Read the model definition and answer for the solid it produces. Units are mm, in the model's axes. A direction names the side the tool comes from. Round coordinates to 2 decimals unless told otherwise and drop trailing zeros. Order: outer loops, then holes, each group sorted by start corner. A loop starts at its lowest first (then second) coordinate and runs counter-clockwise, first axis right, second up. Notation, with made-up numbers: (48.25, 67) -> (68.25, 67) arc R18 ccw to (68.25, 83) -> close; hole circle Ø11 at (-8, 14.5). An arc over 180 degrees is marked (long way). Answer as a JSON object with one key per item and string values. Group by question number.
Item 1: Consider probe 1 along Y at (x, z) = (14, -0.75); probe 2 along X at (y, z) = (-0.25, -14.5); probe 3 along X at (y, z) = (-0.5, 1.75). Determine where each line is inside the solid, lowest interval first. Write a range as from..to.
Item 2: Section D-D, the plane z = -10 is taken. Write down the section's boundary in (x, y).
Item 3: The mould has two halves that part along Z. Classify faces 1 (the flat face through (0, -7.45, 0)), 2 (the flat face through (5, -5, -15.8)), 3 (the flat face through (-0.41, -3.56, -9.54)): pulls with the +Z half, pulls with the -Z half, needs draft (parallel to the pull), parting line crosses it, or undercut.
Item 4: Given P1, Ø0.5, axis at x = 5.5, z = -14.5, coming from the +Y side; P2, Ø9, axis at x = 1.5, z = -7, coming from the -Y side; P3, Ø4.5, axis at x = 1.5, z = -0.5, coming from the -Y side, each flat-ended and moving along its own axis, determine where each tip first touches the part or whether it passes through.
Item 5: For faces 4 (the flat face through (4.7, -5, -15)), 5 (the flat face through (0.1, -6.1, 2.5)), 6 (the cylindrical face through (-8.4, 0.1, -1.5)), determine the directions among +Z, -Z, +X, -X, +Y, -Y from which every point of the face is accessible in a straight line to the end or side of a thin tool.
Item 6: Section C-C, the plane x = 14 is taken. Write down the section's boundary in (y, z), plus the area to 3 significant figures.
Item 7: Section A-A, the plane z = -2.5 is taken. Write down the section's boundary in (x, y), plus the area to 3 significant figures.
Item 8: Section B-B, the plane y = -10 is taken. Write down the section's boundary in (x, z).
from build123d import *

# Parameters (mm, degrees)
SKETCH1_R                = 1.6
BOSS_EXTRUDE1_DEPTH      = 2
BOSS_EXTRUDE2_DEPTH      = 1
BOSS_EXTRUDE2_DEPTH_BACK = 15.2
BOSS_EXTRUDE3_START      = -9.8
BOSS_EXTRUDE3_DEPTH      = 1
BOSS_EXTRUDE4_START      = 5.2
BOSS_EXTRUDE4_DEPTH      = 0.5
BOSS_EXTRUDE6_DEPTH      = 1
SKETCH6_R                = 1
BOSS_EXTRUDE7_DEPTH      = 8.8
FILLET1_R                = 1


with BuildPart() as part:
    # Sketch1 → Boss-Extrude1 (new, symmetric)
    with BuildSketch(Plane.XY):
        with BuildLine():
            Line((-14.4, 7.45), (14.4, 7.45))
            ThreePointArc((14.4, 7.45), (16.521320344, 6.571320344), (17.4, 4.45))
            Line((17.4, 4.45), (17.4, -4.45))
            ThreePointArc((17.4, -4.45), (16.521320344, -6.571320344), (14.4, -7.45))
            Line((14.4, -7.45), (-14.4, -7.45))
            ThreePointArc((-14.4, -7.45), (-16.521320344, -6.571320344), (-17.4, -4.45))
            Line((-17.4, -4.45), (-17.4, 4.45))
            ThreePointArc((-17.4, 4.45), (-16.521320344, 6.571320344), (-14.4, 7.45))
        make_face()
        with Locations((14, 0)):
            Circle(SKETCH1_R, mode=Mode.SUBTRACT)
        with Locations(Location((-14, 0, 0), (0, 0, 180))):
            Circle(SKETCH1_R, mode=Mode.SUBTRACT)
        with BuildLine():
            Line((-4.15, 4.25), (-0.808290377, 4.25))
            Line((-0.808290377, 4.25), (0, 2.85))
            Line((0, 2.85), (0.808290377, 4.25))
            Line((0.808290377, 4.25), (4.15, 4.25))
            ThreePointArc((4.15, 4.25), (8.4, 0), (4.15, -4.25))
            Line((4.15, -4.25), (0.808290377, -4.25))
            Line((0.808290377, -4.25), (0, -2.85))
            Line((0, -2.85), (-0.808290377, -4.25))
            Line((-0.808290377, -4.25), (-4.15, -4.25))
            ThreePointArc((-4.15, -4.25), (-8.4, 0), (-4.15, 4.25))
        make_face(mode=Mode.SUBTRACT)
    extrude(amount=BOSS_EXTRUDE1_DEPTH, both=True)

    # Sketch2 → Boss-Extrude2 (add, two sides: drawn at the far end of the back side and taken through both)
    with BuildSketch(Plane.XY.offset(2).offset(-BOSS_EXTRUDE2_DEPTH_BACK)):
        with BuildLine():
            Line((-4.15, 6.1), (4.15, 6.1))
            ThreePointArc((4.15, 6.1), (10.25, 0), (4.15, -6.1))
            Line((4.15, -6.1), (-4.15, -6.1))
            ThreePointArc((-4.15, -6.1), (-10.25, 0), (-4.15, 6.1))
        make_face()
        with BuildLine():
            Line((0.808290377, 4.25), (0, 2.85))
            Line((0, 2.85), (-0.808290377, 4.25))
            Line((-0.808290377, 4.25), (-4.15, 4.25))
            ThreePointArc((-4.15, 4.25), (-8.4, 0), (-4.15, -4.25))
            Line((-4.15, -4.25), (-0.808290377, -4.25))
            Line((-0.808290377, -4.25), (0, -2.85))
            Line((0, -2.85), (0.808290377, -4.25))
            Line((0.808290377, -4.25), (4.15, -4.25))
            ThreePointArc((4.15, -4.25), (8.4, 0), (4.15, 4.25))
            Line((4.15, 4.25), (0.808290377, 4.25))
        make_face(mode=Mode.SUBTRACT)
    extrude(amount=BOSS_EXTRUDE2_DEPTH + BOSS_EXTRUDE2_DEPTH_BACK)

    # Sketch3 → Boss-Extrude3 (add)
    with BuildSketch(Plane.XY.offset(3).offset(BOSS_EXTRUDE3_START)):
        with BuildLine():
            Line((0.808290377, 4.25), (0, 2.85))
            Line((0, 2.85), (-0.808290377, 4.25))
            Line((-0.808290377, 4.25), (-4.15, 4.25))
            ThreePointArc((-4.15, 4.25), (-8.4, 0), (-4.15, -4.25))
            Line((-4.15, -4.25), (-0.808290377, -4.25))
            Line((-0.808290377, -4.25), (0, -2.85))
            Line((0, -2.85), (0.808290377, -4.25))
            Line((0.808290377, -4.25), (4.15, -4.25))
            ThreePointArc((4.15, -4.25), (8.4, 0), (4.15, 4.25))
            Line((4.15, 4.25), (0.808290377, 4.25))
        make_face()
    extrude(amount=BOSS_EXTRUDE3_DEPTH)



with BuildPart() as body_2:
    # Sketch4 → Boss-Extrude4 (new, symmetric)
    with BuildSketch(Plane(origin=(0, 0, 0), x_dir=(0, 0, -1), z_dir=(1, 0, 0)).offset(BOSS_EXTRUDE4_START)):
        with BuildLine():
            Line((13.2, 1), (15.8, 1))
            Line((15.8, 1), (15.8, -10.62))
            ThreePointArc((15.8, -10.62), (14.8, -11.62), (13.8, -10.62))
            Line((13.8, -10.62), (13.8, -1))
            Line((13.8, -1), (13.2, -1))
            Line((13.2, -1), (13.2, 1))
        make_face()
    boss_extrude4 = extrude(amount=BOSS_EXTRUDE4_DEPTH, both=True)


with BuildPart() as part_1:
    add(part.part)

    add(body_2.part)  # Boss-Extrude6 merges body 2
    # Sketch5 → Boss-Extrude6 (add)
    with BuildSketch(Plane(origin=(0, 0, -13.2), x_dir=(-1, 0, 0), z_dir=(0, 0, -1))):
        with BuildLine():
            Line((4.15, 6.1), (-4.15, 6.1))
            ThreePointArc((-4.15, 6.1), (-10.25, 0), (-4.15, -6.1))
            Line((-4.15, -6.1), (4.15, -6.1))
            ThreePointArc((4.15, -6.1), (10.25, 0), (4.15, 6.1))
        make_face()
    extrude(amount=-BOSS_EXTRUDE6_DEPTH)

    # Mirror2: Boss-Extrude4 across plane
    add(boss_extrude4.mirror(Plane(origin=(0, 0, 0), x_dir=(0, 0, 1), z_dir=(1, 0, 0))))

    # Sketch6 → Boss-Extrude7 (add)
    with BuildSketch(Plane.XY.offset(-5.8)):
        with Locations((-4.3, 0)):
            Circle(SKETCH6_R)
        with Locations(Location((4.3, 0, 0), (0, 0, 180))):
            Circle(SKETCH6_R)
    extrude(amount=BOSS_EXTRUDE7_DEPTH)

    # Fillet1
    fillet1_edges = [part_1.edges().sort_by_distance(p)[0] for p in [
        (-5.3, 0, 3),
        (5.3, 0, 3),
    ]]
    fillet(fillet1_edges, radius=FILLET1_R)


solid = part_1.part
Values found:
{
 "1": {"probe 1": "-7.45..-1.6, 1.6..7.45", "probe 2": "-5.7..-4.7, 4.7..5.7", "probe 3": "-17.4..-15.52, -12.48..-8.37, -5.17..-3.43, 3.43..5.17, 8.37..12.48, 15.52..17.4"},
 "2": {"outline": "(-4.15, -6.1) -> (4.15, -6.1) arc R6.1 ccw to (4.15, 6.1) -> (-4.15, 6.1) arc R6.1 ccw to start; hole (-4.15, -4.25) -> (-0.81, -4.25) -> (0, -2.85) -> (0.81, -4.25) -> (4.15, -4.25) arc R4.25 ccw to (4.15, 4.25) -> (0.81, 4.25) -> (0, 2.85) -> (-0.81, 4.25) -> (-4.15, 4.25) arc R4.25 ccw to start"},
 "3": {"face 1": "needs draft", "face 2": "pulls with the -Z half", "face 3": "undercut"},
 "4": {"P1": "y = 1", "P2": "y = -6.1", "P3": "y = -7.45"},
 "5": {"face 4": "-Z, +Y, -Y", "face 5": "+Z, +X, -X, -Y", "face 6": "+Z"},
 "6": {"outline": "(-7.45, -2) -> (-1.6, -2) -> (-1.6, 2) -> (-7.45, 2) -> close; (1.6, -2) -> (7.45, -2) -> (7.45, 2) -> (1.6, 2) -> close", "area": "46.8 mm2"},
 "7": {"outline": "circle Ø2 at (-4.3, 0); (-4.15, -6.1) -> (4.15, -6.1) arc R6.1 ccw to (4.15, 6.1) -> (-4.15, 6.1) arc R6.1 ccw to start; circle Ø2 at (4.3, 0); hole (-4.15, -4.25) -> (-0.81, -4.25) -> (0, -2.85) -> (0.81, -4.25) -> (4.15, -4.25) arc R4.25 ccw to (4.15, 4.25) -> (0.81, 4.25) -> (0, 2.85) -> (-0.81, 4.25) -> (-4.15, 4.25) arc R4.25 ccw to start", "area": "99.4 mm2"},
 "8": {"outline": "(-5.7, -15.8) -> (-4.7, -15.8) -> (-4.7, -13.8) -> (-5.7, -13.8) -> close; (4.7, -15.8) -> (5.7, -15.8) -> (5.7, -13.8) -> (4.7, -13.8) -> close"}
}
